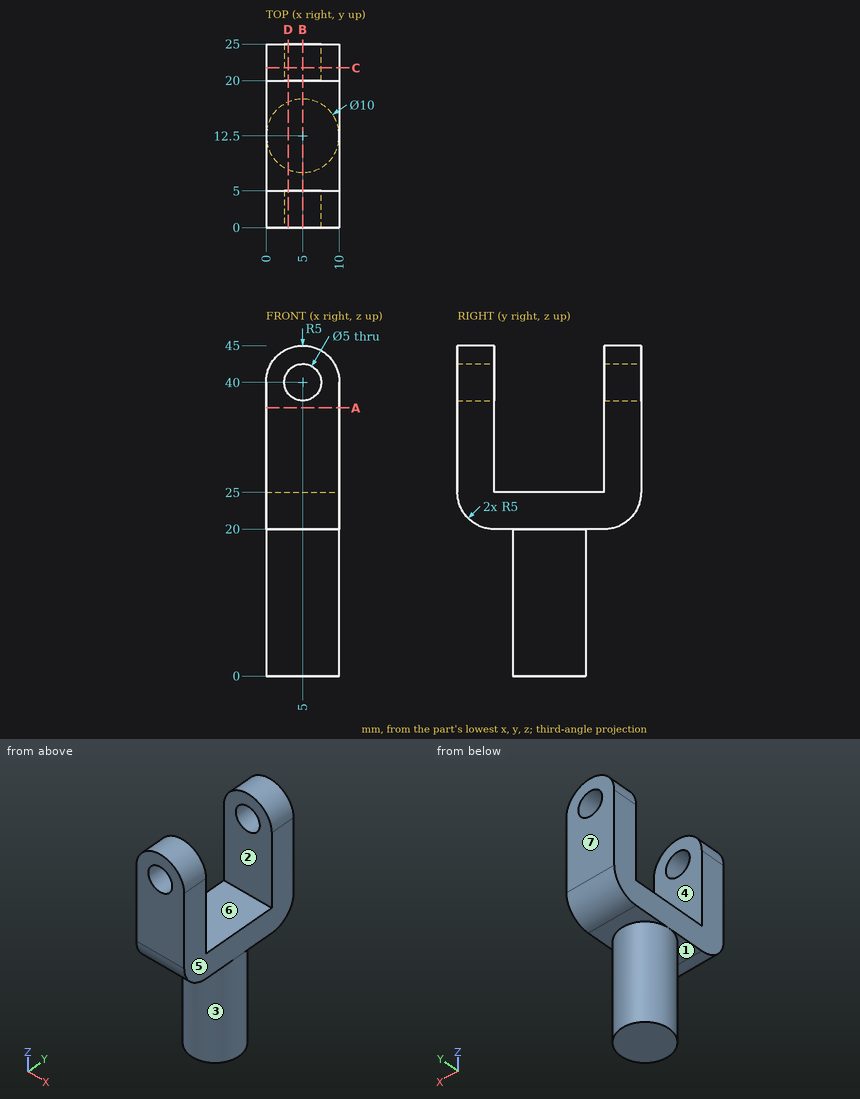
Drawing for the job (mm, zero at the part's lowest x, y, z). A direction names the side the tool comes from. Give positions to 0.01 mm unless a question says otherwise; leave off trailing zeros. Write each loop counter-clockwise with the first axis right and the second up, starting at its lowest first coordinate (ties: lowest second). Pieces come first, ordered by that corner, then holes. Notation, with made-up numbers: (80.25, 61) -> (127.25, 61) arc R4 ccw to (127.25, 65) -> close; hole circle Ø3 at (-7.75, 4). An arc over 180 degrees is marked (long way). Put each result on its own line as item: value. Start each with the question number.
Item 1: Which spindle directions (+Z, -Z, +X, -X, +Y, -Y) get a long thin tool onto all of the face, cutting with end or side? Do the marked faces 1, 2 and 3. Say none if no direction does.
Item 2: Pin check, flat tips, straight feed: pin 1 Ø3 at (x, y) = (6, 12.5) entering from +Z; pin 2 Ø2 at (x, z) = (5, 8) entering from +Y; pin 3 Ø12 at (y, z) = (22.5, 8) entering from -X; pin 4 Ø4.5 at (x, z) = (5, 40) entering from +Y. Stop position of each tip, or through.
Item 3: Cut at D-D (x = 3). List the corners of the cut face in (y, z), then the cut area to 3 significant figures.
Item 4: Cut at A-A (z = 36.5). List the corners of the cut face in (x, y).
Item 5: Pull direction Y, two halves, no side cores. Call the marked faces 4, 5, 6 and 7: pulls with the +Y half, pulls with the -Y half, needs draft (parallel to the pull), parting line crosses it, or undercut.
Item 6: Cut at C-C (y = 21.75). List the corners of the cut face in (x, z), then the cut area to 3 significant figures.
Item 7: Wall check: L1, parallel to Y at x = 3, z = 31.5; L2, parallel to Y at x = 5, z = 19; L3, parallel to Z at x = 7.25, y = 1.25. Give the ranges that are in metal, low to high. Write a range as [from, to].
Item 8: Cut at B-B (x = 5). List the corners of the cut face in (y, z).
Answer list:
1. face 1: -Z, -Y
1. face 2: +Z, +X, -X
1. face 3: -Z
2. pin 1: stops at z = 25
2. pin 2: stops at y = 17.5
2. pin 3: stops at x = 2
2. pin 4: passes through
3. outline: (0, 25) arc R5 ccw to (5, 20) -> (7.92, 20) -> (7.92, 0) -> (17.08, 0) -> (17.08, 20) -> (20, 20) arc R5 ccw to (25, 25) -> (25, 38.5) -> (20, 38.5) -> (20, 25) -> (5, 25) -> (5, 38.5) -> (0, 38.5) -> close; (0, 41.5) -> (5, 41.5) -> (5, 44.58) -> (0, 44.58) -> close; (20, 41.5) -> (25, 41.5) -> (25, 44.58) -> (20, 44.58) -> close
3. area: 463 mm2
4. outline: (0, 0) -> (10, 0) -> (10, 5) -> (0, 5) -> close; (0, 20) -> (10, 20) -> (10, 25) -> (0, 25) -> close
5. face 4: undercut
5. face 5: needs draft
5. face 6: undercut
5. face 7: pulls with the +Y half
6. outline: (0, 20.32) -> (10, 20.32) -> (10, 40) arc R5 ccw to (0, 40) -> close; hole circle Ø5 at (5, 40)
6. area: 216 mm2
7. L1: y = [0, 5], [20, 25]
7. L2: y = [7.5, 17.5]
7. L3: z = [21.69, 38.91], [41.09, 44.47]
8. outline: (0, 25) arc R5 ccw to (5, 20) -> (7.5, 20) -> (7.5, 0) -> (17.5, 0) -> (17.5, 20) -> (20, 20) arc R5 ccw to (25, 25) -> (25, 37.5) -> (20, 37.5) -> (20, 25) -> (5, 25) -> (5, 37.5) -> (0, 37.5) -> close; (0, 42.5) -> (5, 42.5) -> (5, 45) -> (0, 45) -> close; (20, 42.5) -> (25, 42.5) -> (25, 45) -> (20, 45) -> close
